Check sheet for the modelled part. Datum: model origin and axes. Units: mm. Face numbers are marked on the shaded views. A direction names the side the tool comes from. Coordinates: 2 decimals unless noted, no trailing zeros. Loops run counter-clockwise (first coordinate to the right, second up) from the corner with the lowest first, then second, coordinate; pieces in that order, holes last. Notation, with made-up numbers: M 54.25,54.25 L 64.25,54.25 A22 ccw 64.25,61.25 Z; hole C -15,32 d1. An arc over 180 degrees is marked long. Return JSON: item names as keys, results as strings.
from build123d import *

# Parameters (mm, degrees)
SKETCH2_R           = 4
BOSS_EXTRUDE1_DEPTH = 18
SKETCH3_W           = 11.2
SKETCH3_H           = 21.25
SKETCH3_W_2         = 9
SKETCH3_H_2         = 18.05
BOSS_EXTRUDE2_DEPTH = 5
BOSS_EXTRUDE3_START = 19.05
SKETCH4_R           = 3.75
BOSS_EXTRUDE3_DEPTH = 7.5
BOSS_EXTRUDE4_START = -2.2
SKETCH4_3_R         = 1.5
BOSS_EXTRUDE4_DEPTH = 1.5
SKETCH5_R           = 1
CUT_EXTRUDE1_DEPTH  = 1.1
SKETCH6_W           = 2
SKETCH6_H           = 1.25
BOSS_EXTRUDE6_DEPTH = 1


with BuildPart() as part:
    # Sketch2 → Boss-Extrude1 (new body)
    with BuildSketch(Plane(origin=(0, 0, 0), x_dir=(1, 0, 0), z_dir=(0, 1, 0))):
        with Locations(Location((0, 0, 0), (0, 0, 270))):
            Circle(SKETCH2_R)
    extrude(amount=BOSS_EXTRUDE1_DEPTH)

    # Sketch3 → Boss-Extrude2 (add, symmetric)
    with BuildSketch(Plane(origin=(0, 0, 0), x_dir=(0, 0, -1), z_dir=(1, 0, 0))):
        with Locations((0, 8.425)):
            Rectangle(SKETCH3_W, SKETCH3_H)
        with Locations((0, 9.025)):
            Rectangle(SKETCH3_W_2, SKETCH3_H_2, mode=Mode.SUBTRACT)
    extrude(amount=BOSS_EXTRUDE2_DEPTH, both=True)

    # Sketch4 → Boss-Extrude3 (add)
    with BuildSketch(Plane(origin=(0, 0, 0), x_dir=(1, 0, 0), z_dir=(0, 1, 0)).offset(BOSS_EXTRUDE3_START)):
        with Locations(Location((0, 0, 0), (0, 0, 90))):
            Circle(SKETCH4_R)
    extrude(amount=BOSS_EXTRUDE3_DEPTH)

    # Sketch4<3> → Boss-Extrude4 (add)
    with BuildSketch(Plane(origin=(0, 0, 0), x_dir=(1, 0, 0), z_dir=(0, 1, 0)).offset(BOSS_EXTRUDE4_START)):
        with Locations(Location((0, 0, 0), (0, 0, 270))):
            Circle(SKETCH4_3_R)
    extrude(amount=-BOSS_EXTRUDE4_DEPTH)

    # Sketch5 → Cut-Extrude1 (cut)
    with BuildSketch(Plane(origin=(0, 0, -5.6), x_dir=(-1, 0, 0), z_dir=(0, 0, -1))):
        with Locations(Location((-3, 1.3, 0), (0, 0, 90))):
            Circle(SKETCH5_R)
        with Locations(Location((3, 11.3, 0), (0, 0, 90))):
            Circle(SKETCH5_R)
    extrude(amount=-CUT_EXTRUDE1_DEPTH, mode=Mode.SUBTRACT)

    # Sketch6 → Boss-Extrude6 (add)
    with BuildSketch(Plane.XZ.offset(-18.05)):
        Polygon((5, 0), (5, -1.25), (7.5, -1.25), (7.5, 1.25), (5, 1.25), align=None)
        with Locations((4, -0.625)):
            Rectangle(SKETCH6_W, SKETCH6_H)
        with Locations((4, 0.625)):
            Rectangle(SKETCH6_W, SKETCH6_H)
    extrude(amount=BOSS_EXTRUDE6_DEPTH)


solid = part.part
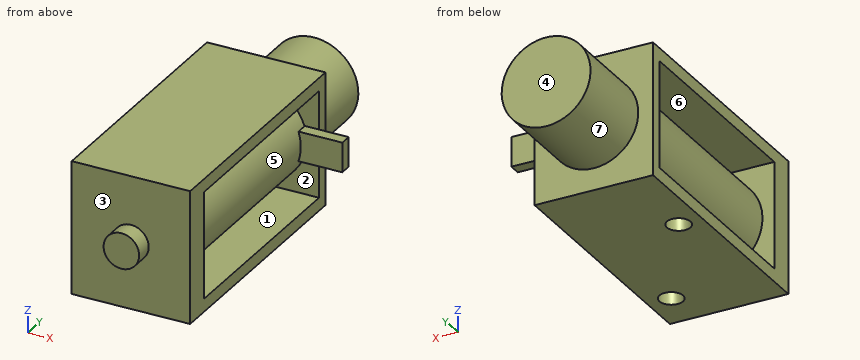
1) Scan lines: line 1 along Z through (x, y) = (0.5, 15); line 2 along Y through (x, z) = (-1, -4); line 3 along Z through (x, y) = (-1.75, 7). Record each from-to range of solid material in increasing order. Write a range as [from, to].
Answers:
{"line 1": "[-5.6, -4.5], [-3.97, 3.97], [4.5, 5.6]", "line 2": "[-2.2, 0], [18.05, 19.05]", "line 3": "[-5.6, -4.5], [-3.6, 3.6], [4.5, 5.6]"}
2) Section check D-D on z = -2. Record the cut outline in (x, y), then the cut area to 3 significant figures.
Answers:
{"outline": "M -5,-2.2 L 5,-2.2 L 5,0 L 3.46,0 L 3.46,18 L -3.46,18 L -3.46,0 L -5,0 Z; M -5,18.05 L 5,18.05 L 5,19.05 L 3.17,19.05 L 3.17,26.55 L -3.17,26.55 L -3.17,19.05 L -5,19.05 Z", "area": "204 mm²"}
3) Draft check along Z on the marked faces 4, 5, 6 and 7. Enter one of: +Z half, -Z half, draft (parallel to the pull), parting line (faces both ways), or undercut.
Answers:
{"face 4": "draft", "face 5": "undercut", "face 6": "undercut", "face 7": "parting line"}
4) Section check C-C on z = 0. Record the cut outline in (x, y).
Answers:
{"outline": "M -5,-2.2 L -1.5,-2.2 L -1.5,-3.7 L 1.5,-3.7 L 1.5,-2.2 L 5,-2.2 L 5,0 L 4,0 L 4,17.05 L 7.5,17.05 L 7.5,18.05 L 5,18.05 L 5,19.05 L 3.75,19.05 L 3.75,26.55 L -3.75,26.55 L -3.75,19.05 L -5,19.05 L -5,18.05 L 3,18.05 L 3,18 L -4,18 L -4,0 L -5,0 Z"}
5) Section check A-A on y = 1.3. Record the cut outline in (x, z).
Answers:
{"outline": "M -5,-5.6 L 2,-5.6 L 2,-4.5 L -5,-4.5 Z; M -5,4.5 L 5,4.5 L 5,5.6 L -5,5.6 Z; C 0,0 d8; M 4,-5.6 L 5,-5.6 L 5,-4.5 L 4,-4.5 Z"}
6) Set-up check for the marked faces 1, 2 and 3: record each of +Z, -Z, +X, -X, +Y, -Y from which the full face is reachable in a straight line by a thin tool's end or side.
Answers:
{"face 1": "+X, -X", "face 2": "-X", "face 3": "-Y"}
7) Go/stop test with flat-tipped pins: pin 1 Ø1 at (x, z) = (3.5, 3.5) entering from +Y; pin 2 Ø5.5 at (y, z) = (13, 0.5) entering from +X; pin 3 Ø2 at (x, z) = (6.5, -0.5) entering from +Y; pin 4 Ø4.5 at (x, z) = (-1.5, -1.5) entering from -Y. Record where each tip stops, or that it passes through.
Answers:
{"pin 1": "y = 19.05", "pin 2": "x = 4", "pin 3": "y = 18.05", "pin 4": "y = -3.7"}
8) Section check B-B on y = 7. Record the cut outline in (x, z), then the cut area to 3 significant figures.
Answers:
{"outline": "M -5,-5.6 L 5,-5.6 L 5,-4.5 L -5,-4.5 Z; M -5,4.5 L 5,4.5 L 5,5.6 L -5,5.6 Z; C 0,0 d8", "area": "72.3 mm²"}
